from build123d import *
from build123d.topology import SkipClean

# Parameters (mm, degrees)
SKETCH1_R           = 3.65
SKETCH1_R_2         = 2.5
BOSS_EXTRUDE1_DEPTH = 4
SKETCH2_R           = 1.25
BOSS_EXTRUDE2_DEPTH = 1.6
CUT_EXTRUDE1_REACH  = 19.71
SKETCH3_R           = 0.5


with BuildPart() as part:
    # Sketch1 → Boss-Extrude1 (new body)
    with BuildSketch(Plane(origin=(0, 0, 0), x_dir=(1, 0, 0), z_dir=(0, 1, 0))):
        with Locations(Location((0, 0, 0), (0, 0, 270))):
            Circle(SKETCH1_R)
        with Locations(Location((0, 0, 0), (0, 0, 270))):
            Circle(SKETCH1_R_2, mode=Mode.SUBTRACT)
    extrude(amount=BOSS_EXTRUDE1_DEPTH)

    # Sketch2 → Boss-Extrude2 (add)
    with SkipClean():  # the faces are left unmerged after this step: merging them gives an invalid solid
        with BuildSketch(Plane(origin=(0, 4, 0), x_dir=(1, 0, 0), z_dir=(0, 1, 0))):
            with BuildLine():
                Line((-2.75, 2.4), (-1.9, 14.5))
                ThreePointArc((-1.9, 14.5), (0, 16.4), (1.9, 14.5))
                Line((1.9, 14.5), (2.75, 2.4))
                ThreePointArc((2.75, 2.4), (0, -3.65), (-2.75, 2.4))
            make_face()
            with Locations(Location((0, 0, 0), (0, 0, 270))):
                Circle(SKETCH2_R, mode=Mode.SUBTRACT)
        extrude(amount=BOSS_EXTRUDE2_DEPTH)
    add(part.part.scale(1), mode=Mode.REPLACE)  # the faces are merged on a copy

    # Sketch3 → Cut-Extrude1 (cut, up to next)
    with BuildSketch(Plane(origin=(0, 5.6, 0), x_dir=(1, 0, 0), z_dir=(0, 1, 0)), mode=Mode.PRIVATE) as cut_extrude1_sk1:
        with Locations(Location((0, 12.5, 0), (0, 0, 270))):
            Circle(SKETCH3_R)
    cut_extrude1_tool1 = extrude(cut_extrude1_sk1.sketch, amount=-CUT_EXTRUDE1_REACH, mode=Mode.PRIVATE) & part.part
    # Sketch3 → Cut-Extrude1 (cut, up to next)
    with BuildSketch(Plane(origin=(0, 5.6, 0), x_dir=(1, 0, 0), z_dir=(0, 1, 0)), mode=Mode.PRIVATE) as cut_extrude1_sk2:
        with Locations(Location((0, 10.5, 0), (0, 0, 270))):
            Circle(SKETCH3_R)
    cut_extrude1_tool2 = extrude(cut_extrude1_sk2.sketch, amount=-CUT_EXTRUDE1_REACH, mode=Mode.PRIVATE) & part.part
    # Sketch3 → Cut-Extrude1 (cut, up to next)
    with BuildSketch(Plane(origin=(0, 5.6, 0), x_dir=(1, 0, 0), z_dir=(0, 1, 0)), mode=Mode.PRIVATE) as cut_extrude1_sk3:
        with Locations(Location((0, 14.5, 0), (0, 0, 270))):
            Circle(SKETCH3_R)
    cut_extrude1_tool3 = extrude(cut_extrude1_sk3.sketch, amount=-CUT_EXTRUDE1_REACH, mode=Mode.PRIVATE) & part.part
    # Sketch3 → Cut-Extrude1 (cut, up to next)
    with BuildSketch(Plane(origin=(0, 5.6, 0), x_dir=(1, 0, 0), z_dir=(0, 1, 0)), mode=Mode.PRIVATE) as cut_extrude1_sk4:
        with Locations(Location((0, 8.5, 0), (0, 0, 270))):
            Circle(SKETCH3_R)
    cut_extrude1_tool4 = extrude(cut_extrude1_sk4.sketch, amount=-CUT_EXTRUDE1_REACH, mode=Mode.PRIVATE) & part.part
    # Sketch3 → Cut-Extrude1 (cut, up to next)
    with BuildSketch(Plane(origin=(0, 5.6, 0), x_dir=(1, 0, 0), z_dir=(0, 1, 0)), mode=Mode.PRIVATE) as cut_extrude1_sk5:
        with Locations(Location((0, 6.5, 0), (0, 0, 270))):
            Circle(SKETCH3_R)
    cut_extrude1_tool5 = extrude(cut_extrude1_sk5.sketch, amount=-CUT_EXTRUDE1_REACH, mode=Mode.PRIVATE) & part.part
    # Sketch3 → Cut-Extrude1 (cut, up to next)
    with BuildSketch(Plane(origin=(0, 5.6, 0), x_dir=(1, 0, 0), z_dir=(0, 1, 0)), mode=Mode.PRIVATE) as cut_extrude1_sk6:
        with Locations(Location((0, 4.5, 0), (0, 0, 270))):
            Circle(SKETCH3_R)
    cut_extrude1_tool6 = extrude(cut_extrude1_sk6.sketch, amount=-CUT_EXTRUDE1_REACH, mode=Mode.PRIVATE) & part.part
    add(cut_extrude1_tool1.solids().sort_by_distance((0, 5.6, -12.5))[0], mode=Mode.SUBTRACT)
    add(cut_extrude1_tool2.solids().sort_by_distance((0, 5.6, -10.5))[0], mode=Mode.SUBTRACT)
    add(cut_extrude1_tool3.solids().sort_by_distance((0, 5.6, -14.5))[0], mode=Mode.SUBTRACT)
    add(cut_extrude1_tool4.solids().sort_by_distance((0, 5.6, -8.5))[0], mode=Mode.SUBTRACT)
    add(cut_extrude1_tool5.solids().sort_by_distance((0, 5.6, -6.5))[0], mode=Mode.SUBTRACT)
    add(cut_extrude1_tool6.solids().sort_by_distance((0, 5.6, -4.5))[0], mode=Mode.SUBTRACT)


solid = part.part
Geometry: final body of the model. Coordinates: model frame, mm. A direction names the side the tool comes from. Give positions to 0.01 mm unless a question says otherwise; leave off trailing zeros. Loops run counter-clockwise (first coordinate to the right, second up) from the corner with the lowest first, then second, coordinate; pieces in that order, holes last. Notation, with made-up numbers: (-35.75, 38) - (1.25, 38) arc R12 cw to (1.25, 50) - close; hole circle Ø4 at (76.5, 35.25). An arc over 180 degrees is marked (long way). Answer as CSV lines item,"result". Start each with the question number.
1. Draft query along X for faces 3 (the face through (0, 5, -13)), 4 (the face through (0, 5, -6)), 5 (the face through (0, 4.8, -16.4)), 6 (the face through (-1, 5.6, -7)). Return one class per face: released by +X, released by -X, zero draft, split by the parting line, or undercut.
2. Ray query, L1, parallel to Y at x = -0.25, z = -5.25; L2, parallel to X at y = 4.95, z = 0; L3, parallel to Z at x = -0.5, y = 1.95. Return the intervals inside material, ascending.
3. Section D-D, the plane y = 0.85. Return loops of the section in (x, z), plus the area to 3 significant figures.
4. Pin query (flat end, axial travel): P1, Ø2, axis at y = 4, z = -11.5, coming from the -X side; P2, Ø2.5, axis at x = 1, z = -0.5, coming from the -Y side. Return the tip coordinate at first contact, or that it passes through.
5. Section A-A, the plane z = -4.5. Return loops of the section in (x, y).
6. Reachability of faces 1 (the face through (-2.44, 1.97, -0.54)), 2 (the face through (0, 5, -5)) from +Z, -Z, +X, -X, +Y, -Y: full face, straight path, thin tool, end or side. Return the list, or none.
7. Section C-C, the plane x = -1. Return loops of the section in (y, z), plus the area to 3 significant figures.
8. Section B-B, the plane y = 4.7. Return loops of the section in (x, z), plus the area to 3 significant figures.
Answers:
1,face 3,"undercut"
1,face 4,"undercut"
1,face 5,"split by the parting line"
1,face 6,"zero draft"
2,L1,"y = 4 to 5.6"
2,L2,"x = -3.65 to -1.25, 1.25 to 3.65"
2,L3,"z = -3.62 to -2.45, 2.45 to 3.62"
3,outline,"circle Ø7.3 at (0, 0); hole circle Ø5 at (0, 0)"
3,area,"22.2 mm2"
4,P1,"stops at x = -2.18"
4,P2,"stops at y = 4"
5,outline,"(-2.6, 4) - (-0.5, 4) - (-0.5, 5.6) - (-2.6, 5.6) - close; (0.5, 4) - (2.6, 4) - (2.6, 5.6) - (0.5, 5.6) - close"
6,face 1,"-Y"
6,face 2,"+Y, -Y"
7,outline,"(0, -3.51) - (4, -3.51) - (4, -16.12) - (5.6, -16.12) - (5.6, -0.75) - (4, -0.75) - (4, -2.29) - (0, -2.29) - close; (0, 2.29) - (4, 2.29) - (4, 0.75) - (5.6, 0.75) - (5.6, 3.51) - (0, 3.51) - close"
7,area,"38.8 mm2"
8,outline,"(-2.75, -2.4) - (-1.9, -14.5) arc R1.9 ccw to (1.9, -14.5) - (2.75, -2.4) arc R3.65 ccw (long way) to start; hole circle Ø2.5 at (0, 0); hole circle Ø1 at (0, -14.5); hole circle Ø1 at (0, -12.5); hole circle Ø1 at (0, -10.5); hole circle Ø1 at (0, -8.5); hole circle Ø1 at (0, -6.5); hole circle Ø1 at (0, -4.5)"
8,area,"89.4 mm2"
